The model under review builds one solid part; all positions refer to its coordinate system, in mm. A direction names the side the tool comes from. Round coordinates to 2 decimals unless told otherwise and drop trailing zeros. Order: outer loops, then holes, each group sorted by start corner. A loop starts at its lowest first (then second) coordinate and runs counter-clockwise, first axis right, second up. Notation, with made-up numbers: M 61,8.5 L 86,8.5 A33 cw 86,36.5 Z; hole C -14,42.5 d4. An arc over 180 degrees is marked long. Answer as CSV lines item,"result". Start each with the question number.
from build123d import *

# Parameters (mm, degrees)
SKETCH1_W                = 64
SKETCH1_H                = 128
BOSS_EXTRUDE1_DEPTH      = 20
BOSS_EXTRUDE2_DEPTH      = 14
BOSS_EXTRUDE3_DEPTH      = 6
BOSS_EXTRUDE3_DEPTH_BACK = 14
SKETCH2_3_R              = 20
SKETCH2_3_R_2            = 10
BOSS_EXTRUDE4_START      = -70
SKETCH4_R                = 20
SKETCH4_R_2              = 10
BOSS_EXTRUDE4_DEPTH      = 20
BOSS_EXTRUDE5_START      = -78
BOSS_EXTRUDE5_DEPTH      = 14
SKETCH8_W                = 64
SKETCH8_H                = 55
CUT_EXTRUDE1_DEPTH       = 8
SKETCH6_W                = 50
SKETCH6_H                = 36
BOSS_EXTRUDE6_DEPTH      = 4
SKETCH7_R                = 7
CUT_EXTRUDE2_DEPTH       = 109.166538264


with BuildPart() as part:
    # Sketch1 → Boss-Extrude1 (new body)
    with BuildSketch(Plane(origin=(0, 0, 0), x_dir=(1, 0, 0), z_dir=(0, 1, 0))):
        Rectangle(SKETCH1_W, SKETCH1_H)
    extrude(amount=BOSS_EXTRUDE1_DEPTH)

    # Sketch2 → Boss-Extrude2 (add)
    with BuildSketch(Plane(origin=(0, 0, -64), x_dir=(-1, 0, 0), z_dir=(0, 0, -1))):
        with BuildLine():
            Line((-19.585841233, 80.049052133), (-32, 20))
            Line((-32, 20), (32, 20))
            Line((32, 20), (19.585841233, 80.049052133))
            ThreePointArc((19.585841233, 80.049052133), (19.8961909, 78.035089105), (20, 76))
            ThreePointArc((20, 76), (-2.035089105, 56.1038091), (-19.585841233, 80.049052133))
        make_face()
    extrude(amount=-BOSS_EXTRUDE2_DEPTH)

    # Sketch2_3 → Boss-Extrude3 (add, two sides: drawn at the far end of the back side and taken through both)
    with BuildSketch(Plane(origin=(0, 0, -64), x_dir=(-1, 0, 0), z_dir=(0, 0, -1)).offset(-BOSS_EXTRUDE3_DEPTH_BACK)):
        with Locations(Location((0, 76, 0), (0, 0, 168.319582439))):
            Circle(SKETCH2_3_R)
        with Locations((0, 76)):
            Circle(SKETCH2_3_R_2, mode=Mode.SUBTRACT)
    extrude(amount=BOSS_EXTRUDE3_DEPTH + BOSS_EXTRUDE3_DEPTH_BACK)



with BuildPart() as body_2:
    # Sketch4 → Boss-Extrude4 (new body)
    with BuildSketch(Plane(origin=(0, 0, -70), x_dir=(-1, 0, 0), z_dir=(0, 0, -1)).offset(BOSS_EXTRUDE4_START)):
        with Locations(Location((0, 76, 0), (0, 0, 168.319582439))):
            Circle(SKETCH4_R)
        with Locations((0, 76)):
            Circle(SKETCH4_R_2, mode=Mode.SUBTRACT)
    extrude(amount=-BOSS_EXTRUDE4_DEPTH)


with BuildPart() as part_1:
    add(part.part)

    add(body_2.part)  # Boss-Extrude5 merges body 2
    # Sketch5 → Boss-Extrude5 (add)
    with BuildSketch(Plane(origin=(0, 0, -64), x_dir=(-1, 0, 0), z_dir=(0, 0, -1)).offset(BOSS_EXTRUDE5_START)):
        with BuildLine():
            Line((32, 20), (19.585841233, 80.049052133))
            ThreePointArc((19.585841233, 80.049052133), (0, 56), (-19.585841233, 80.049052133))
            Line((-19.585841233, 80.049052133), (-32, 20))
            Line((-32, 20), (32, 20))
        make_face()
    extrude(amount=BOSS_EXTRUDE5_DEPTH)

    # Sketch8 → Cut-Extrude1 (cut)
    with BuildSketch(Plane.XZ):
        with Locations((0, -9.5)):
            Rectangle(SKETCH8_W, SKETCH8_H)
    extrude(amount=-CUT_EXTRUDE1_DEPTH, mode=Mode.SUBTRACT)

    # Sketch6 → Boss-Extrude6 (add, symmetric)
    with BuildSketch(Plane(origin=(0, 0, 0), x_dir=(0, 0, -1), z_dir=(1, 0, 0))):
        Polygon((-64, 20), (-14, 20), (-14, 56), align=None)
        with Locations((25, 38)):
            Rectangle(SKETCH6_W, SKETCH6_H)
    extrude(amount=BOSS_EXTRUDE6_DEPTH, both=True)

    # Sketch7 → Cut-Extrude2 (cut, through all)
    with BuildSketch(Plane(origin=(0, 20, 0), x_dir=(1, 0, 0), z_dir=(0, 1, 0))):
        with Locations(Location((18, 16, 0), (0, 0, 270))):
            Circle(SKETCH7_R)
        with Locations(Location((-18, 16, 0), (0, 0, 270))):
            Circle(SKETCH7_R)
        with Locations(Location((18, -43, 0), (0, 0, 270))):
            Circle(SKETCH7_R)
        with Locations(Location((-18, -43, 0), (0, 0, 270))):
            Circle(SKETCH7_R)
    extrude(amount=-CUT_EXTRUDE2_DEPTH, mode=Mode.SUBTRACT)


solid = part_1.part
Item 1: Wall thickness on probe 1 along X at (y, z) = (14, 43); probe 2 along Z at (x, y) = (11.5, 33.5); probe 3 along Z at (x, y) = (13, 62.5): over which ranges is each line inside the solid? List them lowest first. Write a range as [from, to].
Item 2: Consider section C-C (z = 11). State the section outline as (x, y) points, and give its area (3 significant figures).
Item 3: Consider section D-D (x = -23). State the section outline as (y, z) points, and give its area (3 significant figures).
Item 4: Consider section B-B (y = 18). State the section outline as (x, z) points, and give its area (3 significant figures).
Item 5: Consider section A-A (z = 43). State the section outline as (x, y) points.
Item 6: Tool access review of faces 4 (the flat face through (16, 44, 14)), 5 (the flat face through (0, 56, -25)), 6 (the flat face through (0, 4, 18)), 7 (the flat face through (-4, 38, -25)), 8 (the flat face through (18, 20, -25)): name each direction out of +Z, -Z, +X, -X, +Y, -Y from which nothing blocks a thin tool from reaching the whole face with its end or side.
Item 7: For pin 1 (8 mm diameter, centred on x = -23, y = 37.5, fed in from +Z); pin 2 (22.5 mm diameter, centred on x = 20.5, z = -34.5, fed in from +Y); pin 3 (6 mm diameter, centred on y = 53, z = 8, fed in from +X), all flat-tipped, find the tip position at first contact; note any pin that passes through.
Item 8: The part is to be moulded in two halves that separate along X. For faces 1 (the cylindrical face through (1.302, 85.915, 9.86)), 2 (the flat face through (-32, 12, 1)), 3 (the flat face through (0, 0, 41)), say which applies: +X half, -X half, draft (parallel to the pull), parting line (faces both ways), or undercut.
Reported:
1,probe 1,"x = [-32, -25], [-11, 11], [25, 32]"
1,probe 2,"z = [-64, -50], [0, 14]"
1,probe 3,"z = [-70, -50], [0, 20]"
2,outline,"M -32,8 L 32,8 L 32,20 L 19.59,80.05 A20 ccw -19.59,80.05 L -32,20 Z; hole C 0,76 d20"
2,area,"4,020 mm²"
3,outline,"M 0,-64 L 63.53,-64 L 63.53,-50 L 20,-50 L 20,-20.9 L 8,-20.9 L 8,-37 L 0,-37 Z; M 0,18 L 8,18 L 8,-11.1 L 20,-11.1 L 20,0 L 63.53,0 L 63.53,14 L 20,14 L 20,38.1 L 0,38.1 Z; M 0,47.9 L 20,47.9 L 20,64 L 0,64 Z"
3,area,"3,030 mm²"
4,outline,"M -32,-64 L 32,-64 L 32,64 L -32,64 Z; hole C -18,-16 d14; hole C -18,43 d14; hole C 18,-16 d14; hole C 18,43 d14"
4,area,"7,580 mm²"
5,outline,"M -32,0 L -25,0 L -25,20 L -32,20 Z; M -11,0 L 11,0 L 11,20 L 4,20 L 4,35.12 L -4,35.12 L -4,20 L -11,20 Z; M 25,0 L 32,0 L 32,20 L 25,20 Z"
6,face 4,"+Z, +X"
6,face 5,"+X, -X, +Y"
6,face 6,"+X, -X, -Y"
6,face 7,"-X, +Y"
6,face 8,"+X, +Y"
7,pin 1,"stops at z = 14"
7,pin 2,"stops at y = 20"
7,pin 3,"stops at x = 25.8"
8,face 1,"undercut"
8,face 2,"-X half"
8,face 3,"draft"
